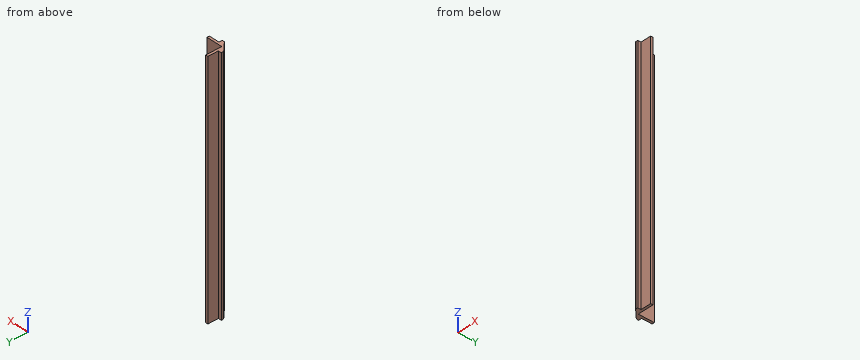
```python
from build123d import *

# Parameters (mm, degrees)
BOSS_EXTRUDE1_DEPTH = 300
FILLET1_R           = 1.5


with BuildPart() as part:
    # Sketch1 → Boss-Extrude1 (new body)
    with BuildSketch(Plane.XY.offset(280)):
        Polygon((-7, 4), (4, -7), (7, -7), (7, -3), (20, -3), (20, 0), (0, 0), (0, 20), (-3, 20), (-3, 7), (-7, 7), align=None)
    extrude(amount=-BOSS_EXTRUDE1_DEPTH)

    # Fillet1
    fillet1_edges = [part.edges().sort_by_distance(p)[0] for p in [
        (4, -7, 130),
        (-7, 4, 130),
    ]]
    fillet(fillet1_edges, radius=FILLET1_R)


solid = part.part
```
Geometry check sheet. Reference: the model listing, model coordinates, mm. Round coordinates to 2 decimals unless told otherwise and drop trailing zeros. Order: outer loops, then holes, each group sorted by start corner. A loop starts at its lowest first (then second) coordinate and runs counter-clockwise, first axis right, second up. Notation, with made-up numbers: (18, 81) - (64, 81) arc R20 ccw to (64, 101) - close; hole circle Ø5 at (86, 85.25). An arc over 180 degrees is marked (long way). Use a Markdown table: item, result. Add a question column.
1) Section check B-B (x = 11.5). Record the cut outline in (y, z), then the cut area to 3 significant figures.
2) Gauge pin test, flat ends, axial feed: P1, Ø16, axis at y = 9, z = 191.5, coming from the +X side; P2, Ø4.5, axis at x = -6, z = 90.5, coming from the +Y side; P3, Ø3, axis at x = 5.5, z = 239.5, coming from the +Y side. Record the tip position at first contact, or that the pin passes through.
3) Thickness scan on line 1 along X through (y, z) = (6, 112); line 2 along Y through (x, z) = (3.5, 3); line 3 along X through (y, z) = (16, 26). Record the ranges inside material, lowest first.
4) Section check A-A (z = 58). Record the cut outline in (x, y).
Established:
| question | item | result |
|---|---|---|
| 1 | outline | (-3, -20) - (0, -20) - (0, 280) - (-3, 280) - close |
| 1 | area | 900 mm2 |
| 2 | P1 | x = 0 |
| 2 | P2 | y = 7 |
| 2 | P3 | y = 0 |
| 3 | line 1 | -7 to 0 |
| 3 | line 2 | -6.5 to 0 |
| 3 | line 3 | -3 to 0 |
| 4 | outline | (-7, 4.62) arc R1.5 ccw to (-6.56, 3.56) - (3.56, -6.56) arc R1.5 ccw to (4.62, -7) - (7, -7) - (7, -3) - (20, -3) - (20, 0) - (0, 0) - (0, 20) - (-3, 20) - (-3, 7) - (-7, 7) - close |
